Autodesk Inventor part; units mm, degrees
ref_plane "YZ Plane" through (0, 0, 0) normal (1, 0, 0) x (0, 1, 0)
ref_plane "XZ Plane" through (0, 0, 0) normal (0, 1, 0) x (-1, 0, 0)
ref_plane "XY Plane" through (0, 0, 0) normal (0, 0, 1) x (1, 0, 0)
sketch "Sketch1" plane through (0, 0, 0) normal (0, 0, 1) x (1, 0, 0)
  line L0 (7.0628, 2) -> (7.0628, -2)
  line L1 (-7.0394, -2) -> (-7.0394, 2)
  line L2 (-7.0394, 2) -> (-4.5826, 2)
  line L3 (4.5826, 2) -> (7.0628, 2)
  line L4 (7.0628, -2) -> (4.5826, -2)
  line L5 (-4.5826, -2) -> (-7.0394, -2)
  arc A0 (-4.5826, -2) -> (4.5826, -2) centre (0, 0) ccw
  arc A1 (4.5826, 2) -> (-4.5826, 2) centre (0, 0) ccw
extrude "Extrusion1" add sketch "Sketch1" along normal blind 20
sketch "Sketch2" plane through (0, 0, 20) normal (0, 0, 1) x (1, 0, 0)
  arc A0 (-1.8, 2.4) -> (1.8, 2.4) centre (0, 0) ccw
  line L0 (-1.8, 2.4) -> (1.8, 2.4)
  dimension "d2" = 6
extrude "Extrusion2" cut sketch "Sketch2" against normal blind 9
sketch "Sketch3" plane through (0, 0, 0) normal (0, 0, -1) x (-1, 0, 0)
  line L0 (2, 2) -> (-2, 2)
  line L1 (-2, 2) -> (-2, -2)
  line L2 (-2, -2) -> (2, -2)
  line L3 (2, -2) -> (2, 2)
  line L4 (2, 2) -> (-2, -2) construction
  line L5 (-2, 2) -> (2, -2) construction
  point P0 (0, 0)
  dimension "d5" = 4
  dimension "d6" = 4
extrude "Extrusion3" cut sketch "Sketch3" against normal blind 9
properties part number "DispenserCoupling"
Could you check a few things on this model? Use its own coordinates, in mm. A direction names the side the tool comes from. Coordinates: 2 decimals unless noted, no trailing zeros. Loops run counter-clockwise (first coordinate to the right, second up) from the corner with the lowest first, then second, coordinate; pieces in that order, holes last.
1. Imagine slicing it at C-C (x = 0). Please give me the cut outline in (y, z).
2. I need wall thicknesses on L1, parallel to X at y = 0.75, z = 7.5; L2, parallel to X at y = 0, z = 18; L3, parallel to Y at x = 6, z = 11. Which ranges of each line are inside material? Lowest first, please.
3. Imagine slicing it at D-D (z = 6). Please give me the cut outline in (x, y), and give its area (3 significant figures).
4. For P1, Ø2.5, axis at x = -6.5, z = 8, coming from the +Y side; P2, Ø5, axis at x = -3.5, z = 9.5, coming from the +Y side; P3, Ø0.7, axis at x = -6, z = 11, coming from the -Y side, each with a flat end and sliding along its axis, tell me the tip position at first contact or that it passes through.
5. Imagine slicing it at A-A (z = 15.25). Please give me the cut outline in (x, y), and give its area (3 significant figures).
6. Imagine slicing it at B-B (y = 0). Please give me the cut outline in (x, z), and give its area (3 significant figures).
7. We'd pull the mould along X, two halves only. Please class faces 4 (the face through (0, -5, 10)), 5 (the face through (0, 2.4, 16)), 6 (the face through (-7.039, 0, 10)): released by +X, released by -X, zero draft, split by the parting line, or undercut.
8. For faces 1 (the face through (-6, -2, 10)), 2 (the face through (6, 2, 10)), 3 (the face through (0, 2, 4)), which set-ups out of +Z, -Z, +X, -X, +Y, -Y let a thin tool reach every point of the face, with its end or its side?
Computed values:
1. outline: (-5, 0) - (-2, 0) - (-2, 9) - (2, 9) - (2, 0) - (5, 0) - (5, 20) - (2.4, 20) - (2.4, 11) - (-3, 11) - (-3, 20) - (-5, 20) - close
2. L1: x = -7.04 to -2, 2 to 7.06
2. L2: x = -7.04 to -3, 3 to 7.06
2. L3: y = -2 to 2
3. outline: (-7.04, -2) - (-4.58, -2) arc R5 ccw to (4.58, -2) - (7.06, -2) - (7.06, 2) - (4.58, 2) arc R5 ccw to (-4.58, 2) - (-7.04, 2) - close; hole (-2, -2) - (2, -2) - (2, 2) - (-2, 2) - close
3. area: 80.0 mm2
4. P1: stops at y = 2
4. P2: stops at y = 4.9
4. P3: stops at y = -2
5. outline: (-7.04, -2) - (-4.58, -2) arc R5 ccw to (4.58, -2) - (7.06, -2) - (7.06, 2) - (4.58, 2) arc R5 ccw to (-4.58, 2) - (-7.04, 2) - close; hole (-1.8, 2.4) arc R3 ccw (long way) to (1.8, 2.4) - close
5. area: 69.2 mm2
6. outline: (-7.04, 0) - (-2, 0) - (-2, 9) - (2, 9) - (2, 0) - (7.06, 0) - (7.06, 20) - (3, 20) - (3, 11) - (-3, 11) - (-3, 20) - (-7.04, 20) - close
6. area: 192 mm2
7. face 4: split by the parting line
7. face 5: undercut
7. face 6: released by -X
8. face 1: +Z, -Z, -X, -Y
8. face 2: +Z, -Z, +X, +Y
8. face 3: -Z
